from build123d import *

# Parameters (mm, degrees)
SKETCH_1_W          = 125
SKETCH_1_H          = 100
SKETCH_1_R          = 1.5
EXTRUDE_1_DEPTH     = 3
SKETCH_2_W          = 110
SKETCH_2_H          = 18
CUT_EXTRUDE_1_DEPTH = 4
SKETCH_3_W          = 125
SKETCH_3_H          = 3
EXTRUDE_2_DEPTH     = 50
SKETCH_4_R          = 1.5
CUT_EXTRUDE_2_DEPTH = 4
FILLET_1_R          = 2


with BuildPart() as part:
    # 草图1 → 凸台-拉伸1 (new body)
    with BuildSketch(Plane.XY):
        with Locations((19.853937426, -18.887566332)):
            Rectangle(SKETCH_1_W, SKETCH_1_H)
        with Locations((-37.096062574, 29.132433668)):
            Circle(SKETCH_1_R, mode=Mode.SUBTRACT)
        with Locations((-23.366062574, 29.132433668)):
            Circle(SKETCH_1_R, mode=Mode.SUBTRACT)
        with Locations((-39.376062574, 13.182433668)):
            Circle(SKETCH_1_R, mode=Mode.SUBTRACT)
        with Locations((-37.096062574, -16.197566332)):
            Circle(SKETCH_1_R, mode=Mode.SUBTRACT)
        with Locations((-37.096062574, -33.707566332)):
            Circle(SKETCH_1_R, mode=Mode.SUBTRACT)
        with Locations((-23.366062574, -33.707566332)):
            Circle(SKETCH_1_R, mode=Mode.SUBTRACT)
        with Locations((56.653937426, 27.572433668)):
            Circle(SKETCH_1_R, mode=Mode.SUBTRACT)
        with Locations((73.063937426, 27.572433668)):
            Circle(SKETCH_1_R, mode=Mode.SUBTRACT)
        with Locations((73.063937426, 15.362433668)):
            Circle(SKETCH_1_R, mode=Mode.SUBTRACT)
        with Locations((29.193937426, -13.557566332)):
            Circle(SKETCH_1_R, mode=Mode.SUBTRACT)
        with Locations((29.193937426, -28.967566332)):
            Circle(SKETCH_1_R, mode=Mode.SUBTRACT)
        with Locations((40.993937426, -28.967566332)):
            Circle(SKETCH_1_R, mode=Mode.SUBTRACT)
        with Locations((26.043937426, -52.367566332)):
            Circle(SKETCH_1_R, mode=Mode.SUBTRACT)
        with Locations((23.833937426, -63.057566332)):
            Circle(SKETCH_1_R, mode=Mode.SUBTRACT)
        with Locations((65.823937426, -60.517566332)):
            Circle(SKETCH_1_R, mode=Mode.SUBTRACT)
        with Locations((78.503937426, -60.517566332)):
            Circle(SKETCH_1_R, mode=Mode.SUBTRACT)
        with Locations((78.503937426, -39.267566332)):
            Circle(SKETCH_1_R, mode=Mode.SUBTRACT)
        with Locations((65.823937426, -38.177566332)):
            Circle(SKETCH_1_R, mode=Mode.SUBTRACT)
        with Locations((-28.646062574, -54.887566332)):
            Circle(SKETCH_1_R, mode=Mode.SUBTRACT)
        with Locations((72.353937426, -10.887566332)):
            Circle(SKETCH_1_R, mode=Mode.SUBTRACT)
        with Locations((12.353937426, 16.112433668)):
            Circle(SKETCH_1_R, mode=Mode.SUBTRACT)
    extrude(amount=EXTRUDE_1_DEPTH)

    # 草图2 → 切除-拉伸1 (cut, through all)
    with BuildSketch(Plane(origin=(0, 0, 0), x_dir=(-1, 0, 0), z_dir=(0, 0, -1))):
        with Locations((-12.353937426, -0.887566332)):
            Rectangle(SKETCH_2_W, SKETCH_2_H)
    extrude(amount=-CUT_EXTRUDE_1_DEPTH, mode=Mode.SUBTRACT)

    # 草图3 → 凸台-拉伸2 (add)
    with BuildSketch(Plane(origin=(0, 31.112433668, 0), x_dir=(1, 0, 0), z_dir=(0, 1, 0))):
        with Locations((19.853937426, -1.5)):
            Rectangle(SKETCH_3_W, SKETCH_3_H)
    extrude(amount=EXTRUDE_2_DEPTH)

    # 草图4 → 切除-拉伸2 (cut, through all)
    with BuildSketch(Plane(origin=(0, 0, 0), x_dir=(-1, 0, 0), z_dir=(0, 0, -1))):
        with Locations((-52.603937426, 68.922433668)):
            Circle(SKETCH_4_R)
        with Locations((22.656062574, 68.922433668)):
            Circle(SKETCH_4_R)
    extrude(amount=-CUT_EXTRUDE_2_DEPTH, mode=Mode.SUBTRACT)

    # 圆角1
    fillet_1_edges = [part.edges().sort_by_distance(p)[0] for p in [
        (-42.646062574, 8.112433668, 1.5),
        (-42.646062574, -9.887566332, 1.5),
        (67.353937426, -9.887566332, 1.5),
        (67.353937426, 8.112433668, 1.5),
        (-42.646062574, 81.112433668, 1.5),
        (82.353937426, 81.112433668, 1.5),
        (82.353937426, -68.887566332, 1.5),
        (-42.646062574, -68.887566332, 1.5),
    ]]
    fillet(fillet_1_edges, radius=FILLET_1_R)


solid = part.part
Design review of the part built by this model. Coordinates are the model's own, in mm. A direction names the side the tool comes from. Coordinates: 2 decimals unless noted, no trailing zeros. Loops run counter-clockwise (first coordinate to the right, second up) from the corner with the lowest first, then second, coordinate; pieces in that order, holes last. Notation, with made-up numbers: (44.25, -6) - (94.25, -6) arc R4 cw to (94.25, -2) - close; hole circle Ø2 at (-24.5, -22). An arc over 180 degrees is marked (long way). Use CSV: the item, a comma, the result in double quotes. Start each with the question number.
1. Add section A-A on x = 60.5. Give the boundary of the cut face in (y, z).
2. Add section B-B on z = 2.5. Count the separate pieces of the cut face and the enclosed holes in it, plus the area to 3 significant figures.
3. To check wall thickness, follow probe 1 along X at (y, z) = (-34, 1.05); probe 2 along Y at (x, z) = (45, 1.2); probe 3 along X at (y, z) = (-5.5, 1.3). State the ranges of each line that lie inside material, in increasing order.
4. Mouldability with a two-part tool opening along X and no side actions: class faces 3 (the flat face through (-42.646, -40, 1)), 4 (the cylindrical face through (-40.875, 13.248, 1.479)), 5 (the flat face through (19, 81.112, 1)) as released by +X, released by -X, zero draft, split by the parting line, or undercut.
5. For faces 1 (the cylindrical face through (-28.971, -56.352, 1.479)), 2 (the flat face through (13, 8.112, 1)), list the 3-axis set-ups (+Z, -Z, +X, -X, +Y, -Y) from which the entire face can be reached by the end or side of a thin tool; tool diameter is ignored.
Resolved:
1,outline,"(-68.89, 0) - (-9.89, 0) - (-9.89, 3) - (-68.89, 3) - close; (8.11, 0) - (81.11, 0) - (81.11, 3) - (8.11, 3) - close"
2,separate pieces,"1"
2,enclosed holes,"23"
2,area,"16,600 mm2"
3,probe 1,"-42.65 to -38.57, -35.62 to -24.84, -21.89 to 82.35"
3,probe 2,"-68.89 to -9.89, 8.11 to 81.11"
3,probe 3,"67.35 to 82.35"
4,face 3,"released by -X"
4,face 4,"undercut"
4,face 5,"zero draft"
5,face 1,"+Z, -Z"
5,face 2,"+Z, -Z, -X"
